For this review, take the finished solid that the model builds, in its own axes (mm). Face numbers are marked on the shaded views. A direction names the side the tool comes from. Coordinates: 2 decimals unless noted, no trailing zeros. Write each loop counter-clockwise with the first axis right and the second up, starting at its lowest first coordinate (ties: lowest second). Pieces come first, ordered by that corner, then holes. Notation, with made-up numbers: (5, 48) - (61, 48) arc R31 cw to (61, 84) - close; hole circle Ø4 at (-31.75, 35). An arc over 180 degrees is marked (long way). Write each question's results on one line, items separated by ' | '.
from build123d import *

# Parameters (mm, degrees)
SKETCH1_W           = 28
SKETCH1_H           = 53
SKETCH1_W_2         = 22
SKETCH1_H_2         = 47
BOSS_EXTRUDE1_DEPTH = 3
SKETCH3_W           = 9.8
SKETCH3_H           = 1.5
BOSS_EXTRUDE2_DEPTH = 1.9
SKETCH4_W           = 16
SKETCH4_H           = 18
CUT_EXTRUDE1_DEPTH  = 57.116040488
FILLET1_R           = 1


with BuildPart() as part:
    # Sketch1 → Boss-Extrude1 (new body)
    # profile 1 of 2: a face of its own
    with BuildSketch(Plane.XY):
        with Locations((11, 23.5)):
            Rectangle(SKETCH1_W, SKETCH1_H)
        with Locations((11, 23.5)):
            Rectangle(SKETCH1_W_2, SKETCH1_H_2, mode=Mode.SUBTRACT)
    # profile 2 of 2: a face of its own
    with BuildSketch(Plane.XY):
        with Locations((11, 23.5)):
            Rectangle(SKETCH1_W_2, SKETCH1_H_2)
    extrude(amount=BOSS_EXTRUDE1_DEPTH)

    # Sketch3 → Boss-Extrude2 (add)
    with BuildSketch(Plane.XY.offset(3)):
        with Locations((11, 47.75)):
            Rectangle(SKETCH3_W, SKETCH3_H)
        with Locations((11, -0.75)):
            Rectangle(SKETCH3_W, SKETCH3_H)
    extrude(amount=BOSS_EXTRUDE2_DEPTH)

    # Sketch4 → Cut-Extrude1 (cut, through all)
    with BuildSketch(Plane(origin=(0, 0, 0), x_dir=(-1, 0, 0), z_dir=(0, 0, -1))):
        with Locations((3, 23.5)):
            Rectangle(SKETCH4_W, SKETCH4_H)
    extrude(amount=-CUT_EXTRUDE1_DEPTH, mode=Mode.SUBTRACT)

    # Fillet1
    fillet1_edges = [part.edges().sort_by_distance(p)[0] for p in [
        (-3, 14.5, 1.5),
        (-3, 32.5, 1.5),
        (5, 14.5, 1.5),
        (5, 32.5, 1.5),
        (-3, -3, 1.5),
        (-3, 50, 1.5),
        (25, 50, 1.5),
        (25, -3, 1.5),
    ]]
    fillet(fillet1_edges, radius=FILLET1_R)


solid = part.part
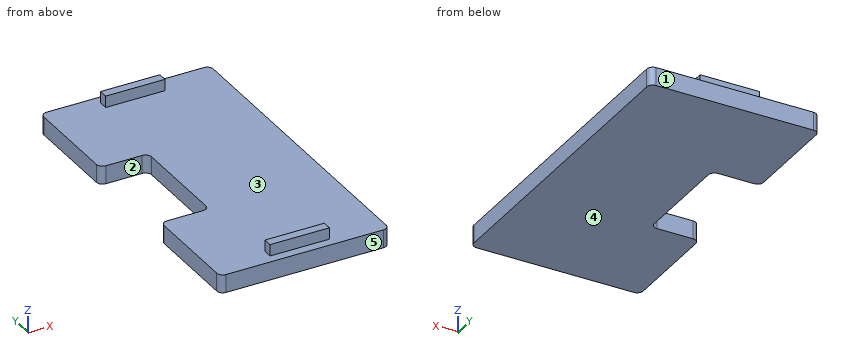
Q1. Wall thickness on line 1 along Z through (x, y) = (-1.25, 3.5); line 2 along Y through (x, z) = (12, 4.45); line 3 along X through (y, z) = (22, 2.5): over which ranges is each line inside the solid? List them lowest first. Write a range as from..to.
Results found:
line 1: 0..3 | line 2: -1.5..0, 47..48.5 | line 3: 5..25
Q2. Take a section at C-C on z = 1.6. State the section outline as (x, y) points.
Results found:
outline: (-3, -2) arc R1 ccw to (-2, -3) - (24, -3) arc R1 ccw to (25, -2) - (25, 49) arc R1 ccw to (24, 50) - (-2, 50) arc R1 ccw to (-3, 49) - (-3, 33.5) arc R1 ccw to (-2, 32.5) - (4, 32.5) arc R1 cw to (5, 31.5) - (5, 15.5) arc R1 cw to (4, 14.5) - (-2, 14.5) arc R1 ccw to (-3, 13.5) - close
Q3. Mouldability with a two-part tool opening along Y and no side actions: class the marked faces 3, 4 and 5 as pulls with the +Y half, pulls with the -Y half, needs draft (parallel to the pull), parting line crosses it, or undercut.
Results found:
face 3: undercut | face 4: needs draft | face 5: pulls with the -Y half
Q4. For the marked faces 1 and 2, list the 3-axis set-ups (+Z, -Z, +X, -X, +Y, -Y) from which the entire face can be reached by the end or side of a thin tool; tool diameter is ignored.
Results found:
face 1: +Z, -Z, +X, -X, +Y | face 2: +Z, -Z, -X
Q5. Take a section at A-A on z = 3.75. State the section outline as (x, y) points.
Results found:
outline: (6.1, -1.5) - (15.9, -1.5) - (15.9, 0) - (6.1, 0) - close; (6.1, 47) - (15.9, 47) - (15.9, 48.5) - (6.1, 48.5) - close
Q6. For pin 1 (2 mm diameter, centred on x = 3, y = 4.5, fed in from +Z); pin 2 (0.8 mm diameter, centred on y = -1, z = 4, fed in from +X); pin 3 (1.6 mm diameter, centred on y = -1, z = 4.5, fed in from -X), all flat-tipped, find the tip position at first contact; note any pin that passes through.
Results found:
pin 1: z = 3 | pin 2: x = 15.9 | pin 3: x = 6.1
Q7. Take a section at D-D on y = 39.5. State the section outline as (x, z) points.
Results found:
outline: (-3, 0) - (25, 0) - (25, 3) - (-3, 3) - close
Q8. Take a section at B-B on x = 9.75. State the section outline as (y, z) points, plus the area to 3 significant figures.
Results found:
outline: (-3, 0) - (50, 0) - (50, 3) - (48.5, 3) - (48.5, 4.9) - (47, 4.9) - (47, 3) - (0, 3) - (0, 4.9) - (-1.5, 4.9) - (-1.5, 3) - (-3, 3) - close | area: 165 mm2
